Input: dimensioned drawing with shaded views. Units: mm. Origin: part minimum x, y, z. A direction names the side the tool comes from. Round coordinates to 2 decimals unless told otherwise and drop trailing zeros. Order: outer loops, then holes, each group sorted by start corner. A loop starts at its lowest first (then second) coordinate and runs counter-clockwise, first axis right, second up. Notation, with made-up numbers: (-34, 27.5) - (25, 27.5) arc R19 cw to (25, 57.5) - close; hole circle Ø2 at (8.5, 18.5). An arc over 180 degrees is marked (long way). Put each result on its own line as item: value. Start each with the question number.
(1) Pin query (flat end, axial travel): P1, Ø0.9, axis at x = 6, y = 6, coming from the +Z side; P2, Ø1.5, axis at x = 37.5, y = 6, coming from the +Z side; P3, Ø2, axis at x = 19, z = 48, coming from the +Y side. Return the tip coordinate at first contact, or that it passes through.
(2) Section D-D (y = 31). Output: boundary loops of the cut face in (x, z).
(3) Section C-C (z = 51.5). Output: boundary loops of the cut face in (x, y), and give its area (3 significant figures).
(4) Access query for the marked faces 1 and 2. Directions: +Z, -Z, +X, -X, +Y, -Y. A direction counts if a zero-diameter tool reaches every point of the face in a straight line with its end or side. Return the directions, or none.
(5) Section B-B (x = 21.15). Output: boundary loops of the cut face in (y, z).
(6) Material intervals for L1, parallel to Y at x = 36.65, z = 38.05; L2, parallel to X at y = 36, z = 37, sorted ascending. Write a range as [from, to].
(7) Section A-A (y = 36.65). Output: boundary loops of the cut face in (x, z), and give its area (3 significant figures).
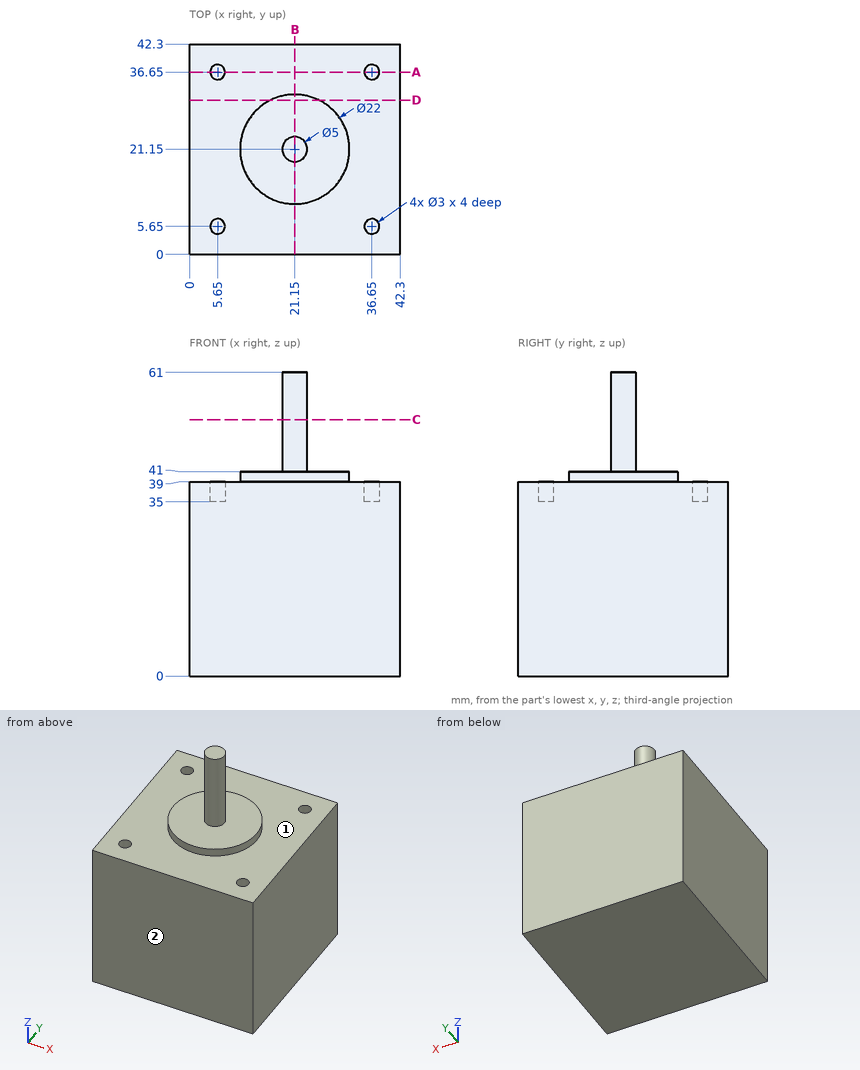
Checks:
1. P1: stops at z = 35
1. P2: stops at z = 39
1. P3: stops at y = 23.37
2. outline: (0, 0) - (42.3, 0) - (42.3, 39) - (26.05, 39) - (26.05, 41) - (16.25, 41) - (16.25, 39) - (0, 39) - close
3. outline: circle Ø5 at (21.15, 21.15)
3. area: 19.6 mm²
4. face 1: +Z
4. face 2: +Z, -Z, +X, -X, -Y
5. outline: (0, 0) - (42.3, 0) - (42.3, 39) - (32.15, 39) - (32.15, 41) - (23.65, 41) - (23.65, 61) - (18.65, 61) - (18.65, 41) - (10.15, 41) - (10.15, 39) - (0, 39) - close
6. L1: y = [0, 4.15], [7.15, 35.15], [38.15, 42.3]
6. L2: x = [0, 4.3], [7, 35.3], [38, 42.3]
7. outline: (0, 0) - (42.3, 0) - (42.3, 39) - (38.15, 39) - (38.15, 35) - (35.15, 35) - (35.15, 39) - (7.15, 39) - (7.15, 35) - (4.15, 35) - (4.15, 39) - (0, 39) - close
7. area: 1,630 mm²
